Autodesk Inventor part; units mm, degrees
ref_plane "YZ Plane" through (0, 0, 0) normal (1, 0, 0) x (0, 1, 0)
ref_plane "XZ Plane" through (0, 0, 0) normal (0, 1, 0) x (-1, 0, 0)
ref_plane "XY Plane" through (0, 0, 0) normal (0, 0, 1) x (1, 0, 0)
sketch "Sketch1" plane through (0, 0, 0) normal (0, 0, 1) x (1, 0, 0)
  line L0 (-40, 40) -> (40, 40)
  line L1 (40, 40) -> (40, -40)
  line L2 (40, -40) -> (-40, -40)
  line L3 (-40, -40) -> (-40, 40)
  point P0 (0, 0)
  dimension "d0" = 80
  dimension "d1" = 80
  dimension "d4" = 40
  dimension "d5" = 40
extrude "Extrusion1" add sketch "Sketch1" along normal blind 8
sketch "Sketch2" plane through (0, 0, 8) normal (0, 0, 1) x (1, 0, 0)
  circle A0 centre (28, 28) radius 2.5
  line L0 (40, 40) -> (-40, 40)
  line L1 (40, -40) -> (40, 40)
  point P0 (0, 0)
  dimension "d6" = 5
  dimension "d7" = 12
  dimension "d8" = 12
extrude "Extrusion2" cut sketch "Sketch2" against normal through all
sketch "Sketch3" plane through (0, 0, 0) normal (0, 0, -1) x (-1, 0, 0)
  circle A0 centre (-28, 28) radius 2.5
  circle A1 centre (-28, 28) radius 8
  point P0 (0, 0)
  dimension "d11" = 16
extrude "Extrusion3" cut sketch "Sketch3" against normal blind 5
sketch "Sketch4" plane through (0, 0, 0) normal (0, 0, -1) x (-1, 0, 0)
  line L0 (40, 40) -> (-40, 40)
  line L1 (9.5, 40) -> (40, 40)
  line L2 (40, 40) -> (40, 9.5)
  line L3 (40, 9.5) -> (9.5, 9.5)
  line L4 (9.5, 9.5) -> (9.5, 40)
  line L5 (40, 40) -> (40, -40)
  point P0 (0, 0)
  dimension "d14" = 30.5
  dimension "d15" = 30.5
  dimension "d16" = 0
extrude "Extrusion4" cut sketch "Sketch4" against normal through all
equation "\"d8\" = d7"
properties part number "top guide support plate"
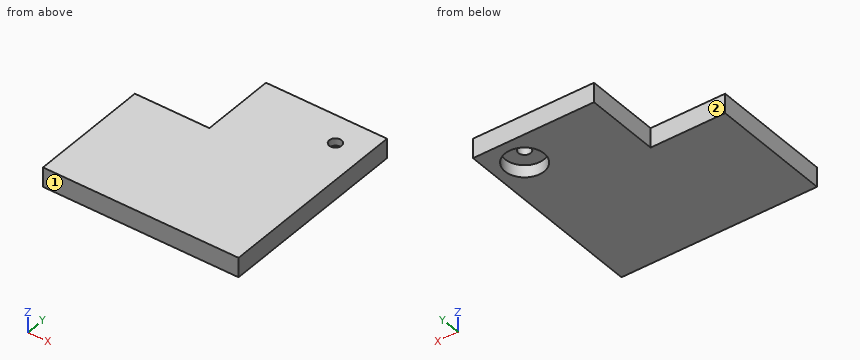
Part model, mm, in its own coordinate system. Face numbers are marked on the shaded views. A direction names the side the tool comes from. Give positions to 0.01 mm unless a question says otherwise; leave off trailing zeros. Write each loop counter-clockwise with the first axis right and the second up, starting at its lowest first coordinate (ties: lowest second). Pieces come first, ordered by that corner, then holes.
1) Which spindle directions (+Z, -Z, +X, -X, +Y, -Y) get a long thin tool onto all of the face, cutting with end or side? Do the marked faces 1 and 2. Say none if no direction does.
Resolved:
face 1: +Z, -Z, +X, -X, -Y
face 2: +Z, -Z, -X, +Y
2) Probe L1, parallel to X at y = 28, z = 6.5; L2, parallel to Y at x = 28, z = 6.05; L3, parallel to Y at x = 28, z = 2.85. List the from-to ranges inside material, lowest first.
Resolved:
L1: x = -9.5 to 25.5, 30.5 to 40
L2: y = -40 to 25.5, 30.5 to 40
L3: y = -40 to 20, 36 to 40
3) Pin check, flat tips, straight feed: pin 1 (13 mm diameter, centred on x = 28, y = 28, fed in from -Z); pin 2 (2.5 mm diameter, centred on x = -19, z = 2.5, fed in from +Y); pin 3 (2.5 mm diameter, centred on y = 26, z = 4.5, fed in from -X). Stop position of each tip, or through.
Resolved:
pin 1: stops at z = 5
pin 2: stops at y = 9.5
pin 3: stops at x = -9.5
4) Cut at A-A on y = 28. Write the cut outline in (x, z).
Resolved:
outline: (-9.5, 0) - (20, 0) - (20, 5) - (25.5, 5) - (25.5, 8) - (-9.5, 8) - close; (30.5, 5) - (36, 5) - (36, 0) - (40, 0) - (40, 8) - (30.5, 8) - close
5) Cut at C-C on z = 6.5. Write the cut outline in (x, y).
Resolved:
outline: (-40, -40) - (40, -40) - (40, 40) - (-9.5, 40) - (-9.5, 9.5) - (-40, 9.5) - close; hole circle Ø5 at (28, 28)
6) Cut at B-B on x = 28. Write the cut outline in (y, z), then the cut area to 3 significant figures.
Resolved:
outline: (-40, 0) - (20, 0) - (20, 5) - (25.5, 5) - (25.5, 8) - (-40, 8) - close; (30.5, 5) - (36, 5) - (36, 0) - (40, 0) - (40, 8) - (30.5, 8) - close
area: 545 mm2
7) Cut at D-D on z = 2.5. Write the cut outline in (x, y).
Resolved:
outline: (-40, -40) - (40, -40) - (40, 40) - (-9.5, 40) - (-9.5, 9.5) - (-40, 9.5) - close; hole circle Ø16 at (28, 28)
